Part print with two shaded views. Sizes in mm from the minimum x, y, z corner. Give positions to 0.01 mm unless a question says otherwise; leave off trailing zeros. Write each loop counter-clockwise with the first axis right and the second up, starting at its lowest first coordinate (ties: lowest second). Pieces come first, ordered by that corner, then holes.
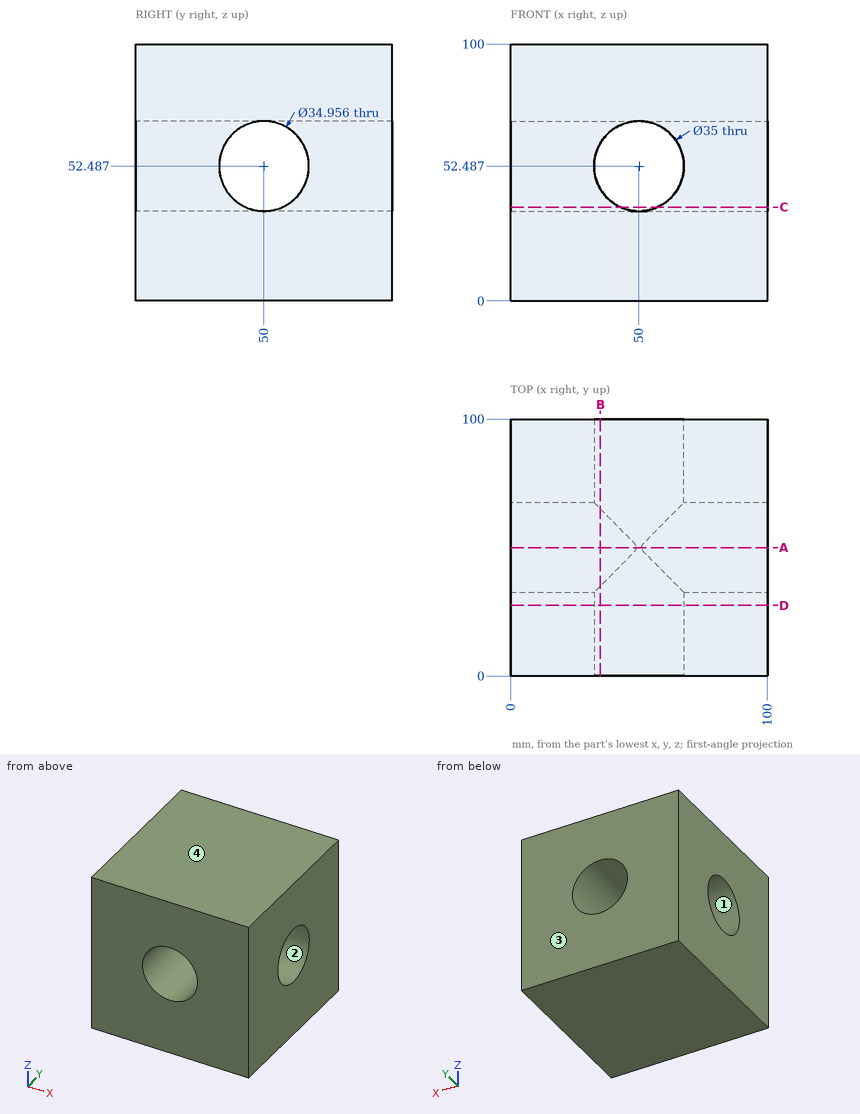
(1) Saw through at B-B, the plane x = 35. List the corners of the cut face in (y, z).
(2) Saw through at D-D, the plane y = 27.5. List the corners of the cut face in (x, z), plus the area to 3 significant figures.
(3) Mould opens along Y. For the marked faces 1, 2, 3 and 4 say: +Y half, -Y half, draft (parallel to the pull), parting line (faces both ways), or undercut.
(4) Saw through at A-A, the plane y = 50. List the corners of the cut face in (x, z) (1 decimal).
(5) Saw through at C-C, the plane z = 36.5. List the corners of the cut face in (x, y).
(6) Probe line 1 (Z direction, x = 50, y = 37.5); line 2 (Z direction, x = 58, y = 89); line 3 (Y direction, x = 67, z = 46). List the from-to ranges inside material, lowest first.
Computed values:
1. outline: (0, 0) - (100, 0) - (100, 43.47) - (64.97, 43.47) arc R17.48 cw to (35.03, 43.47) - (0, 43.47) - close; (0, 61.5) - (35.03, 61.5) arc R17.48 cw to (64.97, 61.5) - (100, 61.5) - (100, 100) - (0, 100) - close
2. outline: (0, 0) - (100, 0) - (100, 100) - (0, 100) - close; hole circle Ø35 at (50, 52.49)
2. area: 9,040 mm2
3. face 1: undercut
3. face 2: undercut
3. face 3: +Y half
3. face 4: draft
4. outline: (0, 0) - (100, 0) - (100, 35) - (50.9, 35) arc R17.5 cw to (49.1, 35) - (0, 35) - close; (0, 70) - (49.1, 70) arc R17.5 cw to (50.9, 70) - (100, 70) - (100, 100) - (0, 100) - close
5. outline: (0, 0) - (42.88, 0) - (42.88, 42.94) - (0, 42.94) - close; (0, 57.06) - (42.88, 57.06) - (42.88, 100) - (0, 100) - close; (57.12, 0) - (100, 0) - (100, 42.94) - (57.12, 42.94) - close; (57.12, 57.06) - (100, 57.06) - (100, 100) - (57.12, 100) - close
6. line 1: z = 0 to 34.99, 69.99 to 100
6. line 2: z = 0 to 36.92, 68.05 to 100
6. line 3: y = 0 to 33.77, 66.23 to 100
